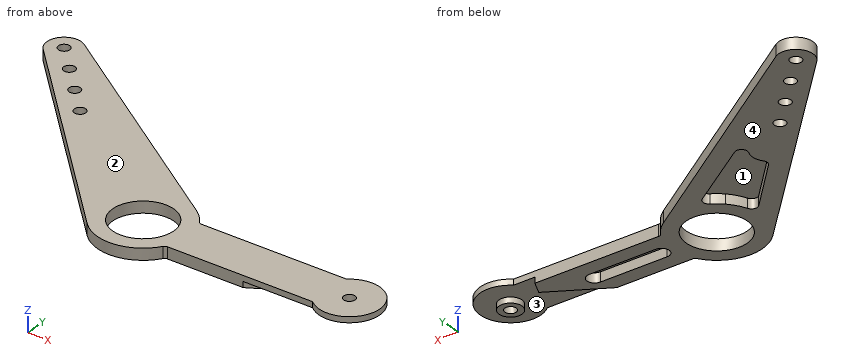
Autodesk Inventor part; units mm, degrees
ref_plane "YZ Plane" through (0, 0, 0) normal (1, 0, 0) x (0, 1, 0)
ref_plane "XZ Plane" through (0, 0, 0) normal (0, 1, 0) x (-1, 0, 0)
ref_plane "XY Plane" through (0, 0, 0) normal (0, 0, 1) x (1, 0, 0)
sketch "スケッチ1" plane through (0, 0, 0) normal (0, 0, 1) x (1, 0, 0)
  circle A0 centre (-55, 0) radius 8.025
  circle A1 centre (-55, 0) radius 12.025
  line L0 (6, -6) -> (-61, -6)
  line L1 (-61, -6) -> (-61, 6)
  line L2 (-61, 6) -> (6, 6)
  line L3 (-61, -6) -> (-61, 6)
  line L4 (-20.8557, 4.9841) -> (202.5072, 4.9841) construction
  circle A2 centre (0, 0) radius 8
  line L5 (-23.9175, 26.3005) -> (3.7655, 4.6721)
  circle A3 centre (0, 0) radius 1.5
  circle A4 centre (0, 0) radius 3
  line L6 (-23.8151, -6) -> (-9.3095, 2.3748)
  line L7 (-9.3095, 2.3748) -> (-11, 6)
  line L8 (-55, 0) -> (0, 0)
  line L9 (0, 0) -> (0, 6)
  line L10 (-55, 0) -> (-112.4533, 48.2091)
  circle A5 centre (-112.4533, 48.2091) radius 4.5
  line L11 (-48.2337, 9.9407) -> (-109.9213, 51.9291)
  line L12 (-115.6772, 45.0695) -> (-63.6148, -8.3897)
  circle A6 centre (-112.4533, 48.2091) radius 1.5
  line L13 (-112.4533, 48.2091) -> (-74.1421, 8.87)
  circle A7 centre (-106.1742, 41.7614) radius 1.5
  circle A8 centre (-99.895, 35.3138) radius 1.5
  circle A9 centre (-93.6158, 28.8662) radius 1.5
  circle A10 centre (-57.5782, 13.277) radius 1.5
  circle A11 centre (-55, 0) radius 11 construction
  circle A12 centre (-57.5782, 13.277) radius 2.5
  point P0 (-62.7295, -9.2117)
  point P1 (-47.2705, 9.2117)
  point P2 (-5.2915, 6)
  point P3 (-5.2915, -6)
  point P4 (-44.5788, 6)
  point P5 (-44.5788, -6)
  point P6 (-49.6708, 6)
  point P7 (-49.6708, -6)
  point P8 (-60.3292, -6)
  point P9 (-61, -5.3292)
  point P10 (-61, 5.3292)
  point P11 (-60.3292, 6)
  point P12 (2.066, 6)
  point P13 (5.2915, -6)
  point P14 (5.2915, 6)
  point P15 (-57.2923, 11.8045)
  point P16 (-56.1715, 15.3437)
  point P17 (-55.4185, 12.0177)
  point P18 (-59.1096, 11.301)
  dimension "d1" = 16.05
  dimension "d3" = 4
  dimension "d19" = 38
  dimension "d35" = 16
  dimension "d36" = 3
  dimension "d37" = 6
  dimension "d38" = 55
  dimension "d39" = 6
  dimension "d40" = 6
  dimension "d42" = 65
  dimension "d43" = 11
  dimension "d44" = 4
  dimension "d45" = 30
  dimension "d47" = 75
  dimension "d50" = 9
  dimension "d51" = 3
  dimension "d54" = 9
  dimension "d59" = 140
  dimension "d63" = 9
  dimension "d67" = 3
  dimension "d68" = 22
  dimension "d69" = 1
extrude "押し出し1" add sketch "スケッチ1" along normal blind 3 contours L8 A1 L0 A0 | A0 L2 A1 L8 | A0 L2 L1 L10 A1 A12 | L0 A1 L10 A0 L1 | L8 L6 L0 A1 | A1 L2 L7 L6 L8 | A0 L1 L2 | L0 L1 A0 | L8 A2 L0 L6 | L6 L7 L2 A2 L8 | A1 A12 L11 | L12 A5 L13 A7 L10 A1 | L8 A4 L9 L2 A2 L0 | A2 L2 L9 A4 L8 | A12 A1 | A10 | A1 A12 | A12 A1 L10 A7 A5 L11 | A2 L5 L2 | A5 L10 A6 L13 | L0 A2 | L8 A3 L9 A4 | A4 L9 A3 L8 | A2 L2 L5 | L13 A6 L10 A5 | A5 L10 A7 L13
extrude "押し出し3" cut sketch "スケッチ1" along normal blind 1.5 contours L8 A2 L0 L6 | L6 L7 L2 A2 L8 | L8 A4 L9 L2 A2 L0 | A2 L2 L9 A4 L8 | A2 L5 L2 | L0 A2 | A2 L2 L5
sketch "スケッチ2" plane through (0, 0, 3) normal (0, 0, 1) x (1, 0, 0)
  circle A0 centre (-55, 0) radius 8.025
  circle A1 centre (0, 0) radius 1.5
  arc A2 (-44.5788, 6) -> (-48.2337, 9.9407) centre (-55, 0) ccw
  line L0 (-48.2337, 9.9407) -> (-109.9213, 51.9291)
  arc A3 (-109.9213, 51.9291) -> (-115.6772, 45.0695) centre (-112.4533, 48.2091) ccw
  line L1 (-115.6772, 45.0695) -> (-63.6148, -8.3897)
  arc A4 (-63.6148, -8.3897) -> (-44.5788, -6) centre (-55, 0) ccw
  line L2 (-44.5788, -6) -> (-5.2915, -6)
  arc A5 (-5.2915, -6) -> (-5.2915, 6) centre (0, 0) ccw
  line L3 (-5.2915, 6) -> (-44.5788, 6)
  circle A6 centre (-112.4533, 48.2091) radius 1.5
  circle A7 centre (-93.6158, 28.8662) radius 1.5
  circle A8 centre (-99.895, 35.3138) radius 1.5
  circle A9 centre (-106.1742, 41.7614) radius 1.5
  dimension "d64" = 9
  dimension "d65" = 9
  dimension "d66" = 9
sketch "スケッチ3" plane through (0, 0, 0) normal (0, 0, -1) x (-1, 0, 0)
  circle A0 centre (106.1742, 41.7614) radius 1.5
  circle A1 centre (99.895, 35.3138) radius 1.5
  circle A2 centre (93.6158, 28.8662) radius 1.5
  circle A3 centre (112.4533, 48.2091) radius 1.5
  line L0 (11, 6) -> (9.3095, 2.3748)
  line L1 (9.3095, 2.3748) -> (23.8151, -6)
  line L2 (44.5788, -6) -> (23.8151, -6)
  arc A4 (44.5788, -6) -> (63.6148, -8.3897) centre (55, 0) ccw
  line L3 (115.6772, 45.0695) -> (63.6148, -8.3897)
  arc A5 (115.6772, 45.0695) -> (109.9213, 51.9291) centre (112.4533, 48.2091) ccw
  line L4 (48.2337, 9.9407) -> (109.9213, 51.9291)
  arc A6 (48.2337, 9.9407) -> (44.5788, 6) centre (55, 0) ccw
  line L5 (11, 6) -> (44.5788, 6)
  circle A7 centre (55, 0) radius 8.025
  arc A8 (78.5193, -24.8633) -> (80.7612, -22.8663) centre (79.3836, -23.5767) ccw
  line L6 (78.5193, -24.8633) -> (60.9226, -13.0433)
  arc A9 (61.0119, -10.4143) -> (60.9226, -13.0433) centre (61.7868, -11.7567) ccw
  arc A10 (61.0119, -10.4143) -> (66.3, -4.1122) centre (55, 0) ccw
  arc A11 (68.8736, -3.5676) -> (66.3, -4.1122) centre (67.7566, -4.6422) ccw
  line L7 (68.8736, -3.5676) -> (80.9904, -16.1632)
  arc A12 (81.1255, -18.1514) -> (80.9904, -16.1632) centre (79.8733, -17.2378) ccw
  arc A13 (81.1255, -18.1514) -> (80.7612, -22.8663) centre (84.7607, -20.8038) ccw
  arc A14 (40.2559, -2) -> (40.2559, 2) centre (40.2559, 0) ccw
  line L8 (40.2559, -2) -> (22.4227, -2)
  arc A15 (22.4227, 2) -> (22.4227, -2) centre (22.4227, 0) ccw
  line L9 (22.4227, 2) -> (40.2559, 2)
  line L10 (9.3095, -2.3748) -> (11, -6)
  line L11 (44.5788, -6) -> (11, -6)
  arc A16 (44.5788, -6) -> (48.2949, -9.9821) centre (55, 0) ccw
  line L12 (102.7709, -46.5745) -> (48.2949, -9.9821)
  arc A17 (102.7709, -46.5745) -> (109.1623, -38.9576) centre (105.5589, -42.424) ccw
  line L13 (63.6661, 8.3366) -> (109.1623, -38.9576)
  arc A18 (63.6661, 8.3366) -> (44.5788, 6) centre (55, 0) ccw
  line L14 (23.8151, 6) -> (44.5788, 6)
  line L15 (23.8151, 6) -> (9.3095, -2.3748)
  circle A19 centre (55, 0) radius 8.025
  circle A20 centre (84.7607, -20.8038) radius 1.5
  circle A21 centre (105.5589, -42.424) radius 1.5
  circle A22 centre (91.6934, -28.0105) radius 1.5
  circle A23 centre (98.6262, -35.2172) radius 1.5
  line L16 (55, 0) -> (46.975, 0)
  arc A24 (80.7612, 22.8663) -> (78.5193, 24.8633) centre (79.3836, 23.5767) ccw
  line L17 (78.5193, 24.8633) -> (60.9226, 13.0433)
  arc A25 (60.9226, 13.0433) -> (61.0119, 10.4143) centre (61.7868, 11.7567) ccw
  arc A26 (66.3, 4.1122) -> (61.0119, 10.4143) centre (55, 0) ccw
  arc A27 (66.3, 4.1122) -> (68.8736, 3.5676) centre (67.7566, 4.6422) ccw
  line L18 (68.8736, 3.5676) -> (80.9904, 16.1632)
  arc A28 (80.9904, 16.1632) -> (81.1255, 18.1514) centre (79.8733, 17.2378) ccw
  arc A29 (80.7612, 22.8663) -> (81.1255, 18.1514) centre (84.7607, 20.8038) ccw
  arc A30 (40.2559, -2) -> (40.2559, 2) centre (40.2559, 0) ccw
  line L19 (40.2559, 2) -> (22.4227, 2)
  arc A31 (22.4227, 2) -> (22.4227, -2) centre (22.4227, 0) ccw
  line L20 (22.4227, -2) -> (40.2559, -2)
  point P0 (0, 0)
  point P1 (0, 0)
  point P2 (61.0119, 10.4143)
extrude "押し出し4" cut sketch "スケッチ3" against normal blind 2.5 contours A25 L17 A24 A29 A28 L18 A27 L13 A18 | L13 A27 A26 | L8 A15 L9 A14
fillet "フィレット2" radius 1 2 edges at (-44.5788, 6, 1.5) (-44.5788, -6, 1.5)
properties part number "アーム中間その弐" material "アルミニウム 7075"
Geometry check sheet. Reference: the model listing, model coordinates, mm. Face numbers are marked on the shaded views. A direction names the side the tool comes from. Round coordinates to 2 decimals unless told otherwise and drop trailing zeros. Order: outer loops, then holes, each group sorted by start corner. A loop starts at its lowest first (then second) coordinate and runs counter-clockwise, first axis right, second up. Notation, with made-up numbers: (8, -10) - (47, -10) arc R30 cw to (47, 27) - close; hole circle Ø10 at (-13.75, -31). An arc over 180 degrees is marked (long way). Use a Markdown table: item, result. Add a question column.
(1) Sectioned sample at D-D, the plane x = -31.5. Enter the section's corners in (y, z).
(2) Tool access check on the marked faces 3 and 4. Record the directions out of +Z, -Z, +X, -X, +Y, -Y that give a thin tool (end or side, any length) a straight path to the whole face; none if there is none.
(3) Sectioned sample at C-C, the plane y = 0. Enter the section's corners in (x, z) (3 decimals), and give its area (3 significant figures).
(4) Depth check by flat-ended pin: pin 1 (1.5 mm diameter, centred on x = -23, z = 2, fed in from +Y); pin 2 (2 mm diameter, centred on x = -36, y = -0.5, fed in from -Z); pin 3 (1.5 mm diameter, centred on y = 25.5, z = 1, fed in from +X). Enter the tip coordinate at first touch or a pass-through.
(5) Material ranges on line 1 along Y through (x, z) = (-23.5, 2.3); line 2 along Y through (x, z) = (0, 1.9); line 3 along Y through (x, z) = (-8, 2.9), recorded low to high. Write a range as [from, to].
(6) Sectioned sample at A-A, the plane x = 0. Enter the section's corners in (y, z), and give its area (3 significant figures).
(7) Sectioned sample at B-B, the plane z = 0.6. Count the separate pieces of the cut face and the enclosed holes in it, and give its area (3 significant figures).
(8) Release check for a two-part mould opening along X. For the marked faces 1 and 2 record: pulls with the +X half, pulls with the -X half, needs draft (parallel to the pull), parting line crosses it, or undercut.
Answers below:
| question | item | result |
|---|---|---|
| 1 | outline | (-6, 0) - (-2, 0) - (-2, 2.5) - (2, 2.5) - (2, 0) - (6, 0) - (6, 3) - (-6, 3) - close |
| 2 | face 3 | -Z |
| 2 | face 4 | -Z, +X, -X, +Y, -Y |
| 3 | outline | (-71.785, 0) - (-63.025, 0) - (-63.025, 3) - (-71.785, 3) - close; (-46.975, 0) - (-42.256, 0) - (-42.256, 2.5) - (-20.423, 2.5) - (-20.423, 0) - (-13.423, 0) - (-13.423, 1.5) - (-3, 1.5) - (-3, 0) - (-1.5, 0) - (-1.5, 3) - (-46.975, 3) - close; (1.5, 0) - (3, 0) - (3, 1.5) - (8, 1.5) - (8, 3) - (1.5, 3) - close |
| 3 | area | 104 mm² |
| 4 | pin 1 | y = 6 |
| 4 | pin 2 | z = 2.5 |
| 4 | pin 3 | x = -69.99 |
| 5 | line 1 | [-6, -2], [2, 6] |
| 5 | line 2 | [-8, -1.5], [1.5, 8] |
| 5 | line 3 | [-6, 6] |
| 6 | outline | (-8, 1.5) - (-3, 1.5) - (-3, 0) - (-1.5, 0) - (-1.5, 3) - (-8, 3) - close; (1.5, 0) - (3, 0) - (3, 1.5) - (8, 1.5) - (8, 3) - (1.5, 3) - close |
| 6 | area | 24.0 mm² |
| 7 | separate pieces | 2 |
| 7 | enclosed holes | 8 |
| 7 | area | 1,330 mm² |
| 8 | face 1 | undercut |
| 8 | face 2 | needs draft |
